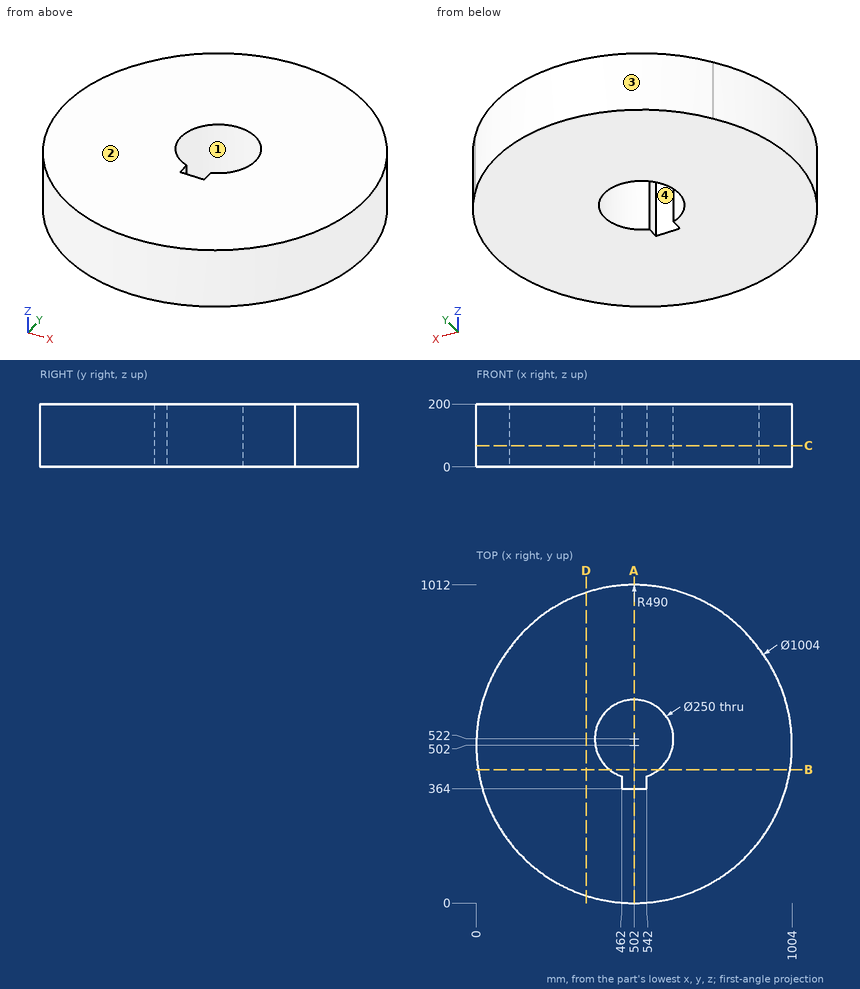
Source: three-view drawing plus pictorial views. Frame: mm from the lowest corner of the part. Round coordinates to 2 decimals unless told otherwise and drop trailing zeros. Write each loop counter-clockwise with the first axis right and the second up, starting at its lowest first coordinate (ties: lowest second). Pieces come first, ordered by that corner, then holes. Notation, with made-up numbers: M 0,-27.75 L 58,-27.75 A22 cw 58,6.25 Z; hole C 66,80 d2. An arc over 180 degrees is marked long. One line per item, written item: value. Start each with the question number.
Item 1: Section query B-B (y = 424.5). Return the cut outline in (x, z), plus the area to 3 significant figures.
Item 2: Section query A-A (x = 502). Return the cut outline in (y, z), plus the area to 3 significant figures.
Item 3: Section query D-D (x = 349). Return the cut outline in (y, z), plus the area to 3 significant figures.
Item 4: Ray query, L1, parallel to Y at x = 502, z = 97; L2, parallel to X at y = 522, z = 59; L3, parallel to X at y = 194.5, z = 11. Return the intervals inside material, ascending. Write a range as from..to.
Item 5: Mould query, pull axis Y, two halves, no side actions, for the marked faces 1, 2, 3 and 4. Classes: pulls with the +Y half, pulls with the -Y half, needs draft (parallel to the pull), parting line crosses it, or undercut.
Item 6: Pin query (flat end, axial travel): pin 1 (1 mm diameter, centred on y = 424, z = 133, fed in from -X); pin 2 (1 mm diameter, centred on x = 336, z = 173.5, fed in from -Y); pin 3 (3 mm diameter, centred on x = 443.5, z = 144, fed in from +Y). Return the tip coordinate at first contact, or that it passes through.
Item 7: Section query C-C (z = 67.5). Return the cut outline in (x, y), plus the area to 3 significant figures.
Result set:
1. outline: M 6.02,0 L 423.78,0 L 423.78,200 L 6.02,200 Z; M 580.22,0 L 997.98,0 L 997.98,200 L 580.22,200 Z
1. area: 167,000 mm²
2. outline: M 0,0 L 364,0 L 364,200 L 0,200 Z; M 647,0 L 1012,0 L 1012,200 L 647,200 Z
2. area: 146,000 mm²
3. outline: M 23.88,0 L 987.5,0 L 987.5,200 L 23.88,200 Z
3. area: 193,000 mm²
4. L1: y = 0..364, 647..1012
4. L2: x = 0.4..377, 627..1003.6
4. L3: x = 105.2..898.8
5. face 1: undercut
5. face 2: needs draft
5. face 3: pulls with the +Y half
5. face 4: undercut
6. pin 1: stops at x = 6.02
6. pin 2: stops at y = 28.07
6. pin 3: stops at y = 1008.67
7. outline: M 105.28,809.6 A502 ccw long 898.72,809.6 A490 ccw Z; hole M 462,364 L 542,364 L 542,403.57 A125 ccw long 462,403.57 Z
7. area: 745,000 mm²
